For this review, take the finished solid that the model builds, in its own axes (mm). A direction names the side the tool comes from. Round coordinates to 2 decimals unless told otherwise and drop trailing zeros. Write each loop counter-clockwise with the first axis right and the second up, starting at its lowest first coordinate (ties: lowest second). Pieces come first, ordered by that corner, then holes.
from build123d import *

# Parameters (mm, degrees)
SKETCH1_R           = 1.6
BOSS_EXTRUDE1_DEPTH = 5
SKETCH3_W           = 45.4
SKETCH3_H           = 34
SKETCH3_R           = 3
BOSS_EXTRUDE2_DEPTH = 3
BOSS_EXTRUDE3_DEPTH = 30
SKETCH5_R           = 3.1
CUT_EXTRUDE2_DEPTH  = 63.178452859
SKETCH6_W           = 45.4
SKETCH6_H           = 38
SKETCH6_R           = 3.1
BOSS_EXTRUDE4_DEPTH = 3.9
SKETCH9_W           = 2.7
SKETCH9_H           = 34
CUT_EXTRUDE3_DEPTH  = 30
CHAMFER1_SIZE       = 2.7


with BuildPart() as part:
    # Sketch1 → Boss-Extrude1 (new body)
    with BuildSketch(Plane.XY):
        Polygon((22.7, 15), (22.7, 19), (-22.7, 19), (-22.7, 15), (-22.7, -15), (22.7, -15), align=None)
        with Locations((-10, 10)):
            Circle(SKETCH1_R, mode=Mode.SUBTRACT)
        with Locations((10, 10)):
            Circle(SKETCH1_R, mode=Mode.SUBTRACT)
        with Locations((10, -10)):
            Circle(SKETCH1_R, mode=Mode.SUBTRACT)
        with Locations((-10, -10)):
            Circle(SKETCH1_R, mode=Mode.SUBTRACT)
    extrude(amount=BOSS_EXTRUDE1_DEPTH)

    # Sketch3 → Boss-Extrude2 (add)
    with BuildSketch(Plane.XY.offset(5)):
        with Locations((0, 2)):
            Rectangle(SKETCH3_W, SKETCH3_H)
        with Locations((10, -10)):
            Circle(SKETCH3_R, mode=Mode.SUBTRACT)
        with Locations((10, 10)):
            Circle(SKETCH3_R, mode=Mode.SUBTRACT)
        with Locations((-10, 10)):
            Circle(SKETCH3_R, mode=Mode.SUBTRACT)
        with Locations((-10, -10)):
            Circle(SKETCH3_R, mode=Mode.SUBTRACT)
    extrude(amount=BOSS_EXTRUDE2_DEPTH)

    # Sketch2 → Boss-Extrude3 (add)
    with BuildSketch(Plane.XY.offset(8)):
        Polygon((15, 15), (15, -15), (22.7, -15), (22.7, 19), (-22.7, 19), (-22.7, -15), (-15, -15), (-15, 15), align=None)
    extrude(amount=BOSS_EXTRUDE3_DEPTH)

    # Sketch5 → Cut-Extrude2 (cut, through all)
    with BuildSketch(Plane(origin=(22.7, 0, 0), x_dir=(0, 0, -1), z_dir=(1, 0, 0))):
        with Locations((-23, 0)):
            Circle(SKETCH5_R)
    extrude(amount=-CUT_EXTRUDE2_DEPTH, mode=Mode.SUBTRACT)

    # Sketch6 → Boss-Extrude4 (add)
    with BuildSketch(Plane(origin=(0, 19, 0), x_dir=(1, 0, 0), z_dir=(0, 1, 0))):
        with Locations((0, 19)):
            Rectangle(SKETCH6_W, SKETCH6_H)
        with Locations(Location((0, 28, 0), (0, 0, 270))):
            Circle(SKETCH6_R, mode=Mode.SUBTRACT)
    extrude(amount=-BOSS_EXTRUDE4_DEPTH)

    # Sketch9 → Cut-Extrude3 (cut)
    with BuildSketch(Plane.XY.offset(38)):
        with Locations((-21.35, 2)):
            Rectangle(SKETCH9_W, SKETCH9_H)
        with Locations((21.35, 2)):
            Rectangle(SKETCH9_W, SKETCH9_H)
    extrude(amount=-CUT_EXTRUDE3_DEPTH, mode=Mode.SUBTRACT)

    # Chamfer1
    chamfer1_edges = [part.edges().sort_by_distance(p)[0] for p in [
        (20, 2, 8),
        (-20, 2, 8),
    ]]
    chamfer(chamfer1_edges, length=CHAMFER1_SIZE - 0.0001)  # a hair under: the kernel refuses the full size


solid = part.part
(1) Mouldability with a two-part tool opening along Y and no side actions: class faces 1 (the face through (0, 19, -1)), 2 (the face through (0, -15, 6)), 3 (the face through (-12.21, -7.97, 6.48)), 4 (the face through (0, 0, 8)) as pulls with the +Y half, pulls with the -Y half, needs draft (parallel to the pull), parting line crosses it, or undercut.
Geometry check:
face 1: pulls with the +Y half
face 2: pulls with the -Y half
face 3: undercut
face 4: needs draft
(2) We need section C-C, the plane y = 0. State how many separate pieces and enclosed holes the cut face has, and give its area (3 significant figures).
Geometry check:
separate pieces: 3
enclosed holes: 0
area: 608 mm2
(3) For line 1 along Y through (x, z) = (10, 3.3); line 2 along Y through (x, z) = (-10, 6.9); line 3 along X through (y, z) = (11, 13), list the stretches that pass through material, from the lowest coordinate up.
Geometry check:
line 1: y = -15 to -11.6, -8.4 to 8.4, 11.6 to 19
line 2: y = -15 to -13, -7 to 7, 13 to 19
line 3: x = -20 to -15, 15 to 20
(4) For faces 5 (the face through (0, 15.1, -19)), 6 (the face through (-20, 2, 28)), 7 (the face through (-8.7, -11.3, 5)), 8 (the face through (-17.5, 0.1, 26.1)), 9 (the face through (20, 2, 28)), list the 3-axis set-ups (+Z, -Z, +X, -X, +Y, -Y) from which the entire face can be reached by the end or side of a thin tool; tool diameter is ignored.
Geometry check:
face 5: -Z, +X, -X, -Y
face 6: +Z, -X, +Y, -Y
face 7: +Z
face 8: +X, -X
face 9: +Z, +X, +Y, -Y
(5) For pin 1 Ø3 at (x, y) = (11, 9) entering from +Z; pin 2 Ø8 at (x, y) = (7, 7) entering from -Z; pin 3 Ø10 at (y, z) = (0, 23) entering from -X; pin 4 Ø10 at (x, z) = (0, -28) entering from +Y, all flat-tipped, find the tip position at first contact; note any pin that passes through.
Geometry check:
pin 1: stops at z = 5
pin 2: stops at z = 0
pin 3: stops at x = -20
pin 4: stops at y = 19
(6) We need section B-B, the plane x = 16. Give the boundary of the cut face in (y, z).
Geometry check:
outline: (-15, 0) - (15.1, 0) - (15.1, -38) - (19, -38) - (19, 38) - (-15, 38) - close; hole circle Ø6.2 at (0, 23)
(7) We need section D-D, the plane z = -28. Give the boundary of the cut face in (x, y), and give its area (3 significant figures).
Geometry check:
outline: (-22.7, 15.1) - (-3.1, 15.1) - (-3.1, 19) - (-22.7, 19) - close; (3.1, 15.1) - (22.7, 15.1) - (22.7, 19) - (3.1, 19) - close
area: 153 mm2
(8) We need section A-A, the plane x = -10. Give the boundary of the cut face in (y, z), and give its area (3 significant figures).
Geometry check:
outline: (-15, 0) - (-11.6, 0) - (-11.6, 5) - (-13, 5) - (-13, 8) - (-15, 8) - close; (-8.4, 0) - (8.4, 0) - (8.4, 5) - (7, 5) - (7, 8) - (-7, 8) - (-7, 5) - (-8.4, 5) - close; (11.6, 0) - (15.1, 0) - (15.1, -38) - (19, -38) - (19, 38) - (15, 38) - (15, 8) - (13, 8) - (13, 5) - (11.6, 5) - close
area: 472 mm2
